Build history of the part. All positions in model axes, mm. Face numbers are marked on the shaded views. A direction names the side the tool comes from. Round coordinates to 2 decimals unless told otherwise and drop trailing zeros. Write each loop counter-clockwise with the first axis right and the second up, starting at its lowest first coordinate (ties: lowest second). Pieces come first, ordered by that corner, then holes. Notation, with made-up numbers: (63, 23) -> (68, 23) arc R24 ccw to (68, 37) -> close; hole circle Ø6 at (-8.5, 51). An arc over 180 degrees is marked (long way). Answer as CSV lines item,"result".
from build123d import *

# Parameters (mm, degrees)
F1_DEPTH = 32
F2_R     = 5
F4_D     = 14
F6_D     = 14


with BuildPart() as f1:
    # F0 (on Front) → F1 (new body)
    with BuildSketch(Plane.XZ):
        Polygon((-52.5, 38), (-27, 0), (27, 0), (52.5, 38), (112.5, 38), (112.5, 44), (49.300583, 44), (23.800583, 6), (-23.800583, 6), (-49.300583, 44), (-112.5, 44), (-112.5, 38), align=None)
    extrude(amount=F1_DEPTH)

    # F2
    f2_edges = [f1.edges().sort_by_distance(p)[0] for p in [
        (-49.300583, -16, 44),
        (-23.800583, -16, 6),
        (23.800583, -16, 6),
        (49.300583, -16, 44),
        (52.5, -16, 38),
        (27, -16, 0),
        (-27, -16, 0),
        (-52.5, -16, 38),
    ]]
    fillet(f2_edges, radius=F2_R)

    # F4 (through all)
    with Locations(Plane.XY.offset(6)):
        with Locations((0, -16)):
            Hole(F4_D / 2)

    # F6 (through all)
    with Locations(Plane.XY.offset(44)):
        with Locations((-82.5, -16), (82.5, -16)):
            Hole(F6_D / 2)


solid = f1.part
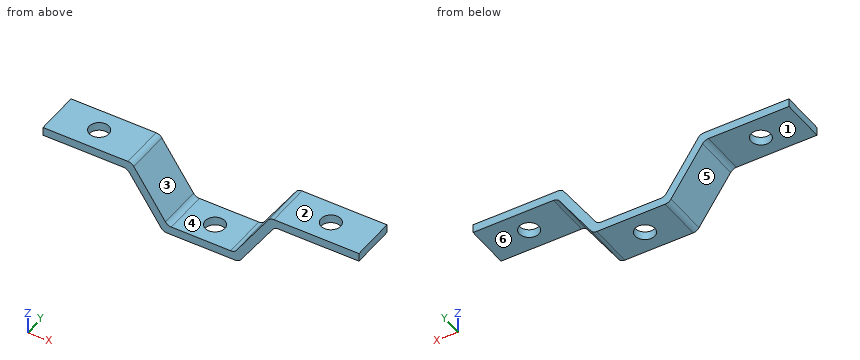
1. Cut at C-C, the plane y = -28.5. Write the cut outline in (x, z).
Results found:
outline,"(-112.5, 38) -> (-55.17, 38) arc R5 cw to (-51.01, 35.79) -> (-28.49, 2.21) arc R5 ccw to (-24.33, 0) -> (24.33, 0) arc R5 ccw to (28.49, 2.21) -> (51.01, 35.79) arc R5 cw to (55.17, 38) -> (112.5, 38) -> (112.5, 44) -> (51.97, 44) arc R5 ccw to (47.81, 41.79) -> (25.29, 8.21) arc R5 cw to (21.13, 6) -> (-21.13, 6) arc R5 cw to (-25.29, 8.21) -> (-47.81, 41.79) arc R5 ccw to (-51.97, 44) -> (-112.5, 44) -> close"
2. Cut at D-D, the plane x = -87. Write the cut outline in (y, z), then the cut area to 3 significant figures.
Results found:
outline,"(-32, 38) -> (-21.36, 38) -> (-21.36, 44) -> (-32, 44) -> close; (-10.64, 38) -> (0, 38) -> (0, 44) -> (-10.64, 44) -> close"
area,"128 mm2"
3. Which spindle directions (+Z, -Z, +X, -X, +Y, -Y) get a long thin tool onto all of the face, cutting with end or side? Do the marked faces 1, 2 and 3. Say none if no direction does.
Results found:
face 1,"-Z, -X, +Y, -Y"
face 2,"+Z, +X, -X, +Y, -Y"
face 3,"+Z, +Y, -Y"
4. Mould opens along X. For the marked faces 4, 5 and 6 say: +X half, -X half, draft (parallel to the pull), parting line (faces both ways), or undercut.
Results found:
face 4,"undercut"
face 5,"-X half"
face 6,"draft"
5. Cut at B-B, the plane y = -16. Count the separate pieces of the cut face and the enclosed holes in it, then the cut area to 3 significant figures.
Results found:
separate pieces,"4"
enclosed holes,"0"
area,"1,340 mm2"
6. Probe line 1 along Y through (x, z) = (82, 40); line 2 along Z through (x, y) = (0.5, -23.5); line 3 along Z through (x, y) = (62.5, -1.5). List the from-to ranges inside material, lowest first.
Results found:
line 1,"y = -32 to -22.98, -9.02 to 0"
line 2,"z = 0 to 6"
line 3,"z = 38 to 44"
7. Drop flat-ended pins along their axis: pin 1 Ø9.5 at (x, y) = (78.5, -12) entering from -Z; pin 2 Ø8 at (y, z) = (-9, 20) entering from +X; pin 3 Ø1 at (x, y) = (24.5, -16) entering from +Z; pin 4 Ø3 at (x, y) = (6.5, -11.5) entering from -Z. Give the stop position or say it passes through.
Results found:
pin 1,"stops at z = 38"
pin 2,"stops at x = 43.11"
pin 3,"stops at z = 7.83"
pin 4,"stops at z = 0"
8. Cut at A-A, the plane x = 0. Write the cut outline in (y, z), then the cut area to 3 significant figures.
Results found:
outline,"(-32, 0) -> (-23, 0) -> (-23, 6) -> (-32, 6) -> close; (-9, 0) -> (0, 0) -> (0, 6) -> (-9, 6) -> close"
area,"108 mm2"
